Part model, mm, in its own coordinate system. A direction names the side the tool comes from. Round coordinates to 2 decimals unless told otherwise and drop trailing zeros. Loops run counter-clockwise (first coordinate to the right, second up) from the corner with the lowest first, then second, coordinate; pieces in that order, holes last. Notation, with made-up numbers: M -40,7 L -35,7 A33 ccw -35,40 Z; hole C 81,-12 d6. An arc over 180 degrees is marked long. Put each result on its own line as item: value. Start each with the question number.
1) Probe line 1 along Y through (x, z) = (32, -13.5) (3 decimals); line 2 along Z through (x, y) = (38.1, 68.45); line 3 along X through (y, z) = (9.5, 5) (3 decimals). List the from-to ranges inside material, lowest first.
2) Pull direction Z, two halves, no side cores. Call faces 3 (the cylindrical face through (49.832, -68.285, -4.864)), 4 (the flat face through (2, -6, 38.1)), 5 (the flat face through (24, -66.675, -1)): +Z half, -Z half, draft (parallel to the pull), parting line (faces both ways), or undercut.
3) Which spindle directions (+Z, -Z, +X, -X, +Y, -Y) get a long thin tool onto all of the face, cutting with end or side? Do faces 1 (the flat face through (24, 66.675, -1)), 2 (the cylindrical face through (49.832, 68.24, -4.864)). Say none if no direction does.
4) Slice it at D-D on z = -32.5. Give the cut face in (x, y) (3 decimals).
5) Slice it at C-C on y = 38. Give the cut face in (x, z) (3 decimals), then the cut area to 3 significant figures.
6) Slice it at A-A on x = 41.5. Give the cut face in (y, z) (3 decimals), then the cut area to 3 significant figures.
7) Drop a flat-ended pin along its axis: pin 1 Ø6 at (y, z) = (-46.5, -6.5) entering from +X (3 decimals). Give the stop position or say it passes through.
8) Slice it at B-B on z = -21. Give the cut face in (x, y) (3 decimals).
```python
from build123d import *

# Parameters (mm, degrees)
F0_W     = 139.7
F0_H     = 76.2
F1_DEPTH = 76.2
F2_W     = 133.35
F2_H     = 76.2
F3_DEPTH = 73.025
F4_R     = 12.7
F5_DEPTH = 171.196


with BuildPart() as f1:
    # F0 (on Right) → F1 (new body)
    with BuildSketch(Plane.YZ):
        Rectangle(F0_W, F0_H)
    extrude(amount=F1_DEPTH)

    # F2 (on face) → F3 (cut)
    with BuildSketch(Plane.YZ.offset(76.2)):
        Rectangle(F2_W, F2_H)
    extrude(amount=-F3_DEPTH, mode=Mode.SUBTRACT)

    # F4 (on face) → F5 (cut)
    with BuildSketch(Plane.XZ.offset(69.85)):
        with BuildLine():
            ThreePointArc((76.2, 0), (65.040768, -26.940768), (38.1, -38.1))
            Line((38.1, -38.1), (76.2, -38.1))
            Line((76.2, -38.1), (76.2, 0))
        make_face()
        with BuildLine():
            ThreePointArc((38.1, 38.1), (65.040768, 26.940768), (76.2, 0))
            Line((76.2, 0), (76.2, 38.1))
            Line((76.2, 38.1), (38.1, 38.1))
        make_face()
        with Locations((38.1, 0)):
            Circle(F4_R)
    extrude(amount=-F5_DEPTH, mode=Mode.SUBTRACT)


solid = f1.part
```
Recorded:
1. line 1: y = -69.85 to -66.675, 66.675 to 69.85
1. line 2: z = -38.1 to -12.7, 12.7 to 38.1
1. line 3: x = 0 to 3.175
2. face 3: undercut
2. face 4: +Z half
2. face 5: draft
3. face 1: +Z, -Z, +X
3. face 2: +Y, -Y
4. outline: M 0,-69.85 L 57.984,-69.85 L 57.984,-66.675 L 3.175,-66.675 L 3.175,66.675 L 57.984,66.675 L 57.984,69.85 L 0,69.85 Z
5. outline: M 0,-38.1 L 3.175,-38.1 L 3.175,38.1 L 0,38.1 Z
5. area: 242 mm2
6. outline: M -69.85,-37.948 L -66.675,-37.948 L -66.675,-12.236 L -69.85,-12.236 Z; M -69.85,12.236 L -66.675,12.236 L -66.675,37.948 L -69.85,37.948 Z; M 66.675,-37.948 L 69.85,-37.948 L 69.85,-12.236 L 66.675,-12.236 Z; M 66.675,12.236 L 69.85,12.236 L 69.85,37.948 L 66.675,37.948 Z
6. area: 327 mm2
7. pin 1: stops at x = 3.175
8. outline: M 0,-69.85 L 69.89,-69.85 L 69.89,-66.675 L 3.175,-66.675 L 3.175,66.675 L 69.89,66.675 L 69.89,69.85 L 0,69.85 Z
